Solid Edge part; units mm, degrees
sketch "Sketch1" plane through (0, 0, 0) normal (1, 0, 0) x (0, 1, 0)
  circle A0 centre (0, 0) radius 4
  circle A1 centre (0, -63.2) radius 4
  line L0 (-15.0147, -31.5995) -> (-15.0147, -6.5995)
  arc A2 (-15.0147, -6.5995) -> (0, 7.9) centre (-0.023, -7.1) cw
  arc A3 (14.9853, -6.2691) -> (0, 7.9) centre (0.0083, -7.1) ccw
  line L1 (14.9853, -6.2691) -> (14.9853, -31.6)
  line L2 (14.9853, -31.6) -> (14.9853, -56.5995)
  arc A4 (-0.023, -71.0991) -> (14.9853, -56.5995) centre (-0.0063, -56.0991) ccw
  arc A5 (-15.0147, -56.5995) -> (-0.023, -71.0991) centre (-0.023, -56.0991) ccw
  line L3 (-15.0147, -56.5995) -> (-15.0147, -31.5995)
extrude "Protrusion1" add sketch "Sketch1" along normal blind 5
sketch "Sketch2" plane through (0, -0.0147, -31.5996) normal (-1, 0, 0) x (0, 0, -1)
  arc A0 (24.9999, 15) -> (24.9999, -15) centre (24.4909, 0) cw
  line L0 (24.9999, -15) -> (24.9999, -12)
  arc A1 (24.9999, 12) -> (24.9999, -12) centre (24.9999, 0) cw
  line L1 (24.9999, 15) -> (24.9999, 12)
extrude "ProtrusiónExtruida_2" add sketch "Sketch2" along normal blind 38
fillet "Redondeo_1" [suppressed]
sketch "Sketch3" plane through (5, -0.0147, -31.5996) normal (1, 0, 0) x (0, 0, -1)
  line L0 (24.9999, -15) -> (24.9999, 15)
  line L1 (24.9999, 15) -> (42.4193, 14.4186)
  line L2 (42.4193, 14.4186) -> (42.4193, -15)
  line L3 (42.4193, -15) -> (24.9999, -15)
extrude "VaciadoExtruido_1" cut sketch "Sketch3" against normal blind 80.5935
sketch "Sketch4" plane through (5, -0.0147, -24.3497) normal (1, 0, 0) x (0, 1, 0)
  line L0 (-15, 17.7502) -> (15.229, 17.7502)
  line L1 (15.229, 17.7502) -> (15.229, 38.738)
  line L2 (15.229, 38.738) -> (-15, 38.738)
  line L3 (-15, 38.738) -> (-15, 17.7502)
extrude "VaciadoExtruido_2" cut sketch "Sketch4" against normal blind 66.5304
sketch "Sketch5" plane through (0, -0.0147, -31.5995) normal (-1, 0, 0) x (0, -1, 0)
  line L0 (-15, 13.9269) -> (12.58, 13.9269)
  line L1 (12.58, 13.9269) -> (12.58, 21.9269)
  line L2 (12.58, 21.9269) -> (-15, 21.9269)
  line L3 (-15, 13.9269) -> (-15, 21.9269)
extrude "ProtrusiónExtruida_4" add sketch "Sketch5" along normal blind 19.3413
sketch "Sketch6" plane through (-9.6707, -12.5947, -13.6726) normal (0, -1, 0) x (1, 0, 0)
  circle A0 centre (-5.0706, 1.2324) radius 2.1262
  circle A1 centre (4.7294, 1.2324) radius 2.125
extrude "VaciadoExtruido_3" cut sketch "Sketch6" against normal blind 36.3882
sketch "Sketch7" plane through (5, -0.0147, -31.5995) normal (1, 0, 0) x (0, -1, 0)
  line L0 (15, 25) -> (-15, 25)
  line L1 (-15, 25) -> (-15, 33)
  line L2 (-15, 33) -> (15, 33)
  line L3 (15, 33) -> (15, 25)
extrude "Protrusion2" add sketch "Sketch7" against normal up to vertex (5 mm away)
sketch "Sketch8" plane through (-7.1707, 14.9853, -35.5995) normal (0, 1, 0) x (1, 0, 0)
  line L0 (-17.1293, -25.9269) -> (-12.1707, -25.9269)
  line L1 (-17.1293, -25.9269) -> (-17.1293, 29)
  line L2 (12.1707, 29) -> (-17.1293, 29)
  line L3 (12.1707, 20.9686) -> (12.1707, 29)
  line L4 (-12.8224, 20.9686) -> (12.1707, 20.9686)
  line L5 (-12.8224, 20.9686) -> (-12.8224, -17.9269)
  line L6 (-12.1707, -17.9269) -> (-12.8224, -17.9269)
  line L7 (-12.1707, -25.9269) -> (-12.1707, -17.9269)
extrude "ProtrusiónExtruida_6" add sketch "Sketch8" against normal blind 27.3963
sketch "Sketch9" plane through (-12.15, -12.411, -37.1361) normal (0, -1, 0) x (-1, 0, 0)
  circle A0 centre (2.59, 24.4635) radius 2.125
  circle A1 centre (-7.21, 24.4635) radius 2.125
extrude "VaciadoExtruido_4" cut sketch "Sketch9" against normal blind 76.7204
sketch "Sketch10" plane through (0, -0.0147, -35.5995) normal (-1, 0, 0) x (0, 0, -1)
  line L0 (-29, -15) -> (-25.9269, -15)
  line L1 (-25.9269, -15) -> (-25.9269, 15)
  line L2 (-25.9269, 15) -> (-29, 15)
  line L3 (-29, 15) -> (-29, -15)
extrude "VaciadoExtruido_5" cut sketch "Sketch10" against normal blind 44.1991
sketch "Sketch11" plane through (2.5, -15.0147, -37.1361) normal (0, -1, 0) x (0, 0, -1)
  line L0 (-27.4635, 2.5) -> (27.4635, 2.5)
  line L1 (27.4635, 2.5) -> (27.4635, 1.5)
  line L2 (27.4635, 1.5) -> (-27.4635, 1.5)
  line L3 (-27.4635, 1.5) -> (-27.4635, 2.5)
  line L4 (27.4635, -26.8) -> (-27.4635, -26.8)
  line L5 (-27.4635, -26.8) -> (-27.4635, -25.8)
  line L6 (-27.4635, -25.8) -> (27.4635, -25.8)
  line L7 (27.4635, -25.8) -> (27.4635, -26.8)
extrude "VaciadoExtruido_6" cut sketch "Sketch11" against normal blind 65.6283
fillet "Redondeo_2" radius 4 4 edges at (-23.3, 1.2871, -64.5995) (4, -0.0147, -64.5995) (-23.3, 1.2871, -9.6726) (4, -0.0147, -9.6726)
sketch "Sketch12" plane through (-9.65, 1.2871, -64.5995) normal (0, 0, -1) x (1, 0, 0)
  circle A0 centre (0, 0) radius 4
extrude "ProtrusiónExtruida_7" add sketch "Sketch12" along normal blind 92.7
fillet "Redondeo_3" radius 4 1 edges at (-13.65, 1.2871, -157.2995)
fillet "Redondeo_4" radius 8 1 edges at (-13.65, 1.2871, -64.5995)
properties material "Aluminum Alloy:3.0505 , AlMn0.5Mg0.6,  EN-AW 3105"
Could you check a few things on this model? Use its own coordinates, in mm. A direction names the side the tool comes from. Coordinates: 2 decimals unless noted, no trailing zeros. Order: outer loops, then holes, each group sorted by start corner. A loop starts at its lowest first (then second) coordinate and runs counter-clockwise, first axis right, second up. Notation, with made-up numbers: (7, 6) -> (41, 6) arc R13 ccw to (41, 24) -> close; hole circle Ø3 at (72, 65). An arc over 180 degrees is marked (long way). One line per item, written item: value. Start each with the question number.
1) Imagine slicing it at B-B on z = -143.5. List the corners of the cut face in (x, y) for me.
2) I'm going to push flat-ended pins straight in: pin 1 (8 mm diameter, centred on x = -12, z = -111, fed in from -Y); pin 2 (2 mm diameter, centred on y = 6, z = -130, fed in from -X); pin 3 (4 mm diameter, centred on x = -8.5, z = -122, fed in from +Y); pin 4 (8 mm diameter, centred on x = -15, z = -42.5, fed in from +Y). Where does each tip first touch, or does it pass through?
3) Which directions (+Z, -Z, +X, -X, +Y, -Y) give clear straight access to the entire face, cutting with the end or side of a thin tool? Please do faces 1 (the flat face through (-21, -12.411, -45)), 2 (the flat face through (-10, 1, -17.673)), 3 (the flat face through (-10, 14, -64.6)).
4) If I drill on L1, parallel to X at y = 6.5, z = -42; L2, parallel to Z at x = -13.75, y = 11.5; L3, parallel to Z at x = 0.5, y = 5, over which ranges is the centre line in solid material (lowest first)? Write a range as [from, to].
5) Imagine slicing it at A-A on z = -19. List the corners of the cut face in (x, y) for me.
6) We'd pull the mould along Z, two halves only. Please class faces 4 (the flat face through (-10, 1, -56.568)), 5 (the cylindrical face through (2.859, 0.195, -63.397)), 6 (the cylindrical face through (-22.159, 1.388, -10.875)): +Z half, -Z half, draft (parallel to the pull), parting line (faces both ways), or undercut.
7) Imagine slicing it at C-C on x = -15.5. Count the separate pieces of the cut face and the enclosed holes in it, plus the area to 3 significant figures.
Answer list:
1. outline: circle Ø8 at (-9.65, 1.29)
2. pin 1: stops at y = -2.71
2. pin 2: stops at x = -11.14
2. pin 3: stops at y = 5.29
2. pin 4: passes through
3. face 1: -Z, -X, -Y
3. face 2: +Y, -Y
3. face 3: -Z, +Y
4. L1: x = [-23.3, -19.99], [0, 4]
4. L2: z = [-64.66, -63.48], [-59.72, -56.57], [-17.67, -14.32], [-10.56, -9.67]
4. L3: z = [-64.57, -9.7]
5. outline: (-23.3, -12.41) -> (-19.99, -12.41) -> (-19.99, 14.99) -> (-23.3, 14.99) -> close; (0, -15.01) -> (4, -15.01) -> (4, 14.99) -> (0, 14.99) -> close
6. face 4: undercut
6. face 5: -Z half
6. face 6: +Z half
7. separate pieces: 4
7. enclosed holes: 0
7. area: 249 mm2
